Geometry check sheet. Reference: the model listing, model coordinates, mm. Round coordinates to 2 decimals unless told otherwise and drop trailing zeros. Write each loop counter-clockwise with the first axis right and the second up, starting at its lowest first coordinate (ties: lowest second). Pieces come first, ordered by that corner, then holes. Notation, with made-up numbers: M -17,74.25 L 10,74.25 A16 ccw 10,79.25 Z; hole C -15,-21.75 d3. An arc over 180 degrees is marked long. Use a Markdown table: item, result.
```python
from build123d import *

# Parameters (mm, degrees)
SKETCH_1_W      = 24
SKETCH_1_H      = 18
SKETCH_1_R      = 1.075
EXTRUDE_1_DEPTH = 2
FILLET_1_R      = 3
FILLET_2_R      = 3
FILLET_3_R      = 3
FILLET_4_R      = 3


with BuildPart() as part:
    # 草图1 → 凸台-拉伸1 (new body)
    with BuildSketch(Plane.XY):
        with Locations((12, -9)):
            Rectangle(SKETCH_1_W, SKETCH_1_H)
        with Locations((21, -3)):
            Circle(SKETCH_1_R, mode=Mode.SUBTRACT)
        with Locations((6, -3)):
            Circle(SKETCH_1_R, mode=Mode.SUBTRACT)
    extrude(amount=EXTRUDE_1_DEPTH)

    # 圆角1
    fillet_1_edges = [part.edges().sort_by_distance(p)[0] for p in [
        (24, 0, 1),
    ]]
    fillet(fillet_1_edges, radius=FILLET_1_R)

    # 圆角2
    fillet_2_edges = [part.edges().sort_by_distance(p)[0] for p in [
        (0, 0, 1),
    ]]
    fillet(fillet_2_edges, radius=FILLET_2_R)

    # 圆角3
    fillet_3_edges = [part.edges().sort_by_distance(p)[0] for p in [
        (0, -18, 1),
    ]]
    fillet(fillet_3_edges, radius=FILLET_3_R)

    # 圆角4
    fillet_4_edges = [part.edges().sort_by_distance(p)[0] for p in [
        (24, -18, 1),
    ]]
    fillet(fillet_4_edges, radius=FILLET_4_R)


solid = part.part
```
Item 1: Cross-section at A-A, the plane x = 6. Record the cut outline in (y, z) (3 decimals), and give its area (3 significant figures).
Outcome:
| item | result |
|---|---|
| outline | M -18,0 L -4.075,0 L -4.075,2 L -18,2 Z; M -1.925,0 L 0,0 L 0,2 L -1.925,2 Z |
| area | 31.7 mm2 |
Item 2: Material ranges on line 1 along Y through (x, z) = (6, 0.65) (3 decimals); line 2 along Y through (x, z) = (5.25, 1.1); line 3 along X through (y, z) = (-1.5, 0.3), recorded low to high. Write a range as from..to.
Outcome:
| item | result |
|---|---|
| line 1 | y = -18..-4.075, -1.925..0 |
| line 2 | y = -18..-3.77, -2.23..0 |
| line 3 | x = 0.4..23.6 |
Item 3: Mould release check, pull along Y, two halves, no side actions. Record for faces 1 (the face through (22.025, -2.677, 0.986)), 2 (the face through (12, -9, 2)), 3 (the face through (12, 0, 1)): +Y half, -Y half, draft (parallel to the pull), parting line (faces both ways), or undercut.
Outcome:
| item | result |
|---|---|
| face 1 | undercut |
| face 2 | draft |
| face 3 | +Y half |
Item 4: Cross-section at C-C, the plane y = -3.5. Record the cut outline in (x, z).
Outcome:
| item | result |
|---|---|
| outline | M 0,0 L 5.05,0 L 5.05,2 L 0,2 Z; M 6.95,0 L 20.05,0 L 20.05,2 L 6.95,2 Z; M 21.95,0 L 24,0 L 24,2 L 21.95,2 Z |
Item 5: Cross-section at B-B, the plane z = 0.55. Record the cut outline in (x, y) (3 decimals), and give its area (3 significant figures).
Outcome:
| item | result |
|---|---|
| outline | M 0,-15 A3 ccw 3,-18 L 21,-18 A3 ccw 24,-15 L 24,-3 A3 ccw 21,0 L 3,0 A3 ccw 0,-3 Z; hole C 6,-3 d2.15; hole C 21,-3 d2.15 |
| area | 417 mm2 |
Item 6: Cross-section at D-D, the plane x = 22.5. Record the cut outline in (y, z), and give its area (3 significant figures).
Outcome:
| item | result |
|---|---|
| outline | M -17.6,0 L -0.4,0 L -0.4,2 L -17.6,2 Z |
| area | 34.4 mm2 |
